```python
from build123d import *

# Parameters (mm, degrees)
SKETCH1_R            = 3.3782
BOSS_EXTRUDE1_DEPTH  = 3.175
BOSS_EXTRUDE2_DEPTH  = 4.445
SKETCH7_W            = 18.542
SKETCH7_H            = 15.24
BOSS_EXTRUDE4_DEPTH  = 8.43915
SKETCH8_R            = 1.4605
CUT_EXTRUDE3_DEPTH   = 21.955
SKETCH9_R            = 10.16
CUT_EXTRUDE4_DEPTH   = 21.955
CUT_EXTRUDE6_DEPTH   = 9.525
SKETCH23_R           = 4.490128061
CUT_EXTRUDE7_DEPTH   = 6.35
BOSS_EXTRUDE10_DEPTH = 3.175
BOSS_EXTRUDE11_DEPTH = 3.175
SKETCH19_W           = 8.382
SKETCH19_H           = 4.445
BOSS_EXTRUDE12_DEPTH = 20.32
BOSS_EXTRUDE13_DEPTH = 4.445
CUT_EXTRUDE5_DEPTH   = 12.7
FILLET2_R            = 3.175


with BuildPart() as part:
    # Sketch1 → Boss-Extrude1 (new body)
    with BuildSketch(Plane(origin=(0, 0, 0), x_dir=(1, 0, 0), z_dir=(0, 1, 0))):
        with BuildLine():
            Line((0, -13.335), (25.4, -13.335))
            Line((25.4, -13.335), (25.4, 13.335))
            Line((25.4, 13.335), (0, 13.335))
            ThreePointArc((0, 13.335), (-13.335, 0), (0, -13.335))
        make_face()
        Circle(SKETCH1_R, mode=Mode.SUBTRACT)
    boss_extrude1 = extrude(amount=BOSS_EXTRUDE1_DEPTH)

    # Sketch2 → Boss-Extrude2 (add)
    with BuildSketch(Plane(origin=(0, 0, 0), x_dir=(-1, 0, 0), z_dir=(0, -1, 0))):
        Polygon((-25.4, 13.335), (-25.4, -13.335), (-13.335, -13.335), (-13.335, 0), (-13.335, 13.335), align=None)
    extrude(amount=BOSS_EXTRUDE2_DEPTH)

    # Mirror2: Boss-Extrude1 across plane
    add(boss_extrude1.mirror(Plane(origin=(0, -2.2225, 0), x_dir=(0, 0, 1), z_dir=(0, -1, 0))))

    # Sketch7 → Boss-Extrude4 (add)
    with BuildSketch(Plane(origin=(0, -7.62, 0), x_dir=(-1, 0, 0), z_dir=(0, -1, 0))):
        with Locations((-16.129, 0)):
            Rectangle(SKETCH7_W, SKETCH7_H)
    extrude(amount=BOSS_EXTRUDE4_DEPTH)

    # Sketch8 → Cut-Extrude3 (cut, through all)
    with BuildSketch(Plane(origin=(0, 0, -7.62), x_dir=(-1, 0, 0), z_dir=(0, 0, -1))):
        with Locations((-20.7645, -12.1285)):
            Circle(SKETCH8_R)
        with Locations((-11.4935, -12.1285)):
            Circle(SKETCH8_R)
    extrude(amount=-CUT_EXTRUDE3_DEPTH, mode=Mode.SUBTRACT)

    # Sketch9 → Cut-Extrude4 (cut, through all)
    with BuildSketch(Plane(origin=(0, 0, -7.62), x_dir=(-1, 0, 0), z_dir=(0, 0, -1))):
        with Locations((-16.129, -23.67915)):
            Circle(SKETCH9_R)
    extrude(amount=-CUT_EXTRUDE4_DEPTH, mode=Mode.SUBTRACT)

    # Sketch22 → Cut-Extrude6 (cut)
    with BuildSketch(Plane(origin=(0, 3.175, 0), x_dir=(1, 0, 0), z_dir=(0, 1, 0))):
        Polygon((19.3675, -4.490128061), (23.857563833, 0.024016226), (19.3675, 4.490128061), (14.877436167, -0.024016226), align=None)
    extrude(amount=-CUT_EXTRUDE6_DEPTH, mode=Mode.SUBTRACT)

    # Sketch23 → Cut-Extrude7 (cut)
    with BuildSketch(Plane(origin=(0, -6.35, 0), x_dir=(1, 0, 0), z_dir=(0, 1, 0))):
        with Locations((19.3675, 0)):
            Circle(SKETCH23_R)
    extrude(amount=CUT_EXTRUDE7_DEPTH, mode=Mode.SUBTRACT)

    # Sketch16 → Boss-Extrude10 (add)
    with BuildSketch(Plane(origin=(0, 3.175, 0), x_dir=(1, 0, 0), z_dir=(0, 1, 0))):
        Polygon((0, 13.335), (-13.335, 13.335), (-13.335, 0), (-13.335, -13.335), (0, -13.335), (-6.6675, -6.6675), (-6.6675, 6.6675), align=None)
    extrude(amount=-BOSS_EXTRUDE10_DEPTH)

    # Sketch17 → Boss-Extrude11 (add)
    with BuildSketch(Plane.XZ.offset(7.62)):
        Polygon((-13.335, -13.335), (-13.335, 0), (-13.335, 13.335), (0, 13.335), (-6.6675, 6.6675), (-6.6675, -6.6675), (0, -13.335), align=None)
    extrude(amount=-BOSS_EXTRUDE11_DEPTH)

    # Sketch19 → Boss-Extrude12 (add)
    with BuildSketch(Plane(origin=(0, 3.175, 0), x_dir=(1, 0, 0), z_dir=(0, 1, 0))):
        with Locations((-2.5019, 11.1125)):
            Rectangle(SKETCH19_W, SKETCH19_H)
    extrude(amount=BOSS_EXTRUDE12_DEPTH)

    # Sketch20 → Boss-Extrude13 (add)
    with BuildSketch(Plane.XY.offset(-8.89)):
        Polygon((-6.6929, 23.495), (-13.335, 3.175), (-6.6929, 3.175), align=None)
    extrude(amount=-BOSS_EXTRUDE13_DEPTH)

    # Sketch21 → Cut-Extrude5 (cut)
    with BuildSketch(Plane.XY.offset(-8.89)):
        Polygon((0, 22.225), (1.6891, 21.610217877), (1.6891, 20.299782123), (0, 19.685), align=None)
    extrude(amount=-CUT_EXTRUDE5_DEPTH, mode=Mode.SUBTRACT)

    # Fillet2
    fillet2_edges = [part.edges().sort_by_distance(p)[0] for p in [
        (-13.335, 1.5875, 13.335),
        (-13.335, -6.0325, 13.335),
    ]]
    fillet(fillet2_edges, radius=FILLET2_R)


solid = part.part
```
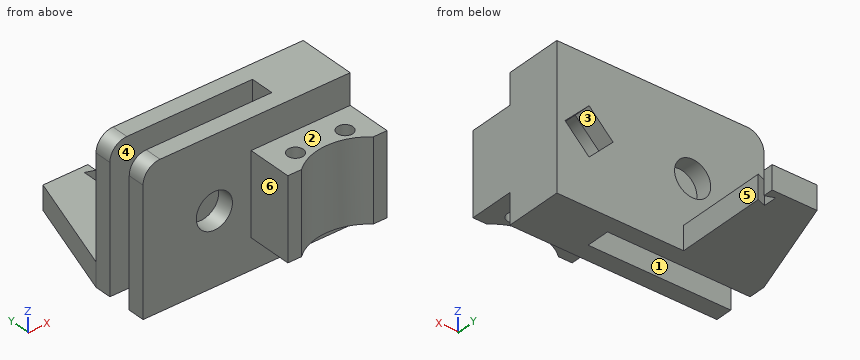
Geometry check sheet. Reference: the model listing, model coordinates, mm. Face numbers are marked on the shaded views. A direction names the side the tool comes from. Round coordinates to 2 decimals unless told otherwise and drop trailing zeros. Write each loop counter-clockwise with the first axis right and the second up, starting at its lowest first coordinate (ties: lowest second). Pieces come first, ordered by that corner, then holes. Notation, with made-up numbers: (88, 34) -> (144, 34) arc R23 cw to (144, 54) -> close; hole circle Ø10 at (72, 46). An arc over 180 degrees is marked (long way). Put each result on its own line as item: value.
1) Thickness scan on probe 1 along X at (y, z) = (-6.05, 0) (3 decimals); probe 2 along Z at (x, y) = (0, -6.85) (3 decimals); probe 3 along Y at (x, z) = (-7.5, 4.5) (3 decimals). Record the ranges inside material, lowest first. Write a range as from..to.
Recorded:
probe 1: x = -13.335..-3.378, 3.378..14.877, 23.858..25.4
probe 2: z = -13.335..-3.378, 3.378..13.335
probe 3: y = -7.62..-4.445, 0..3.175
2) Release check for a two-part mould opening along Z. For the marked faces 1, 2 and 3 record: pulls with the +Z half, pulls with the -Z half, needs draft (parallel to the pull), parting line crosses it, or undercut.
Recorded:
face 1: needs draft
face 2: pulls with the +Z half
face 3: undercut
3) Cross-section at C-C, the plane x = -1.5. Enter the section's corners in (y, z) (3 decimals).
Recorded:
outline: (-7.62, -13.335) -> (-4.445, -13.335) -> (-4.445, -3.027) -> (-7.62, -3.027) -> close; (-7.62, 3.027) -> (-4.445, 3.027) -> (-4.445, 13.335) -> (-7.62, 13.335) -> close; (0, -13.335) -> (23.495, -13.335) -> (23.495, -8.89) -> (3.175, -8.89) -> (3.175, -3.027) -> (0, -3.027) -> close; (0, 3.027) -> (3.175, 3.027) -> (3.175, 13.335) -> (0, 13.335) -> close
4) Cross-section at D-D, the plane y = 2. Give the number of separate pieces and of enclosed holes in the cut face, plus the area to 3 significant figures.
Recorded:
separate pieces: 1
enclosed holes: 2
area: 955 mm2
5) Depth check by flat-ended pin: P1, Ø11, axis at x = 0, z = 0, coming from the +Y side (3 decimals); P2, Ø9.5, axis at x = 16, y = -10.5, coming from the +Z side (3 decimals); P3, Ø2, axis at y = 10, z = -12, coming from the +X side; P4, Ø6, axis at x = 4, y = -11, coming from the -Z side. Enter the tip coordinate at first touch or a pass-through.
Recorded:
P1: stops at y = 3.175
P2: stops at z = 13.335
P3: stops at x = 1.69
P4: stops at z = -7.62
6) Cross-section at A-A, the plane x = 11. Enter the section's corners in (y, z) (3 decimals).
Recorded:
outline: (-14.909, -7.62) -> (-13.503, -7.62) -> (-13.503, 7.62) -> (-14.909, 7.62) -> close; (-10.754, -7.62) -> (-7.62, -7.62) -> (-7.62, -13.335) -> (-4.445, -13.335) -> (-4.445, 13.335) -> (-7.62, 13.335) -> (-7.62, 7.62) -> (-10.754, 7.62) -> close; (0, -13.335) -> (3.175, -13.335) -> (3.175, 13.335) -> (0, 13.335) -> close
7) Access from +Z, -Z, +X, -X, +Y, -Y to the whole of each face (thin tool, end or side, straight path). Record for the marked faces 4, 5 and 6.
Recorded:
face 4: +Z, -Z, -X
face 5: +Z, -Z, +X, +Y
face 6: +Z, -Z, -X, -Y
8) Cross-section at B-B, the plane y = -11.5. Enter the section's corners in (x, z).
Recorded:
outline: (6.86, -7.62) -> (10.18, -7.62) -> (10.18, 7.62) -> (6.86, 7.62) -> close; (12.81, -7.62) -> (19.45, -7.62) -> (19.45, 7.62) -> (12.81, 7.62) -> close; (22.08, -7.62) -> (25.4, -7.62) -> (25.4, 7.62) -> (22.08, 7.62) -> close
